Source: three-view drawing plus pictorial views. Frame: mm from the lowest corner of the part. Coordinates: 2 decimals unless noted, no trailing zeros. Write each loop counter-clockwise with the first axis right and the second up, starting at its lowest first coordinate (ties: lowest second). Pieces come first, ordered by that corner, then holes. Notation, with made-up numbers: (-25.5, 51.5) -> (23.5, 51.5) arc R19 ccw to (23.5, 69.5) -> close; hole circle Ø8 at (-27, 85.5). An arc over 180 degrees is marked (long way). One line per item, written item: value. Start each with the question number.
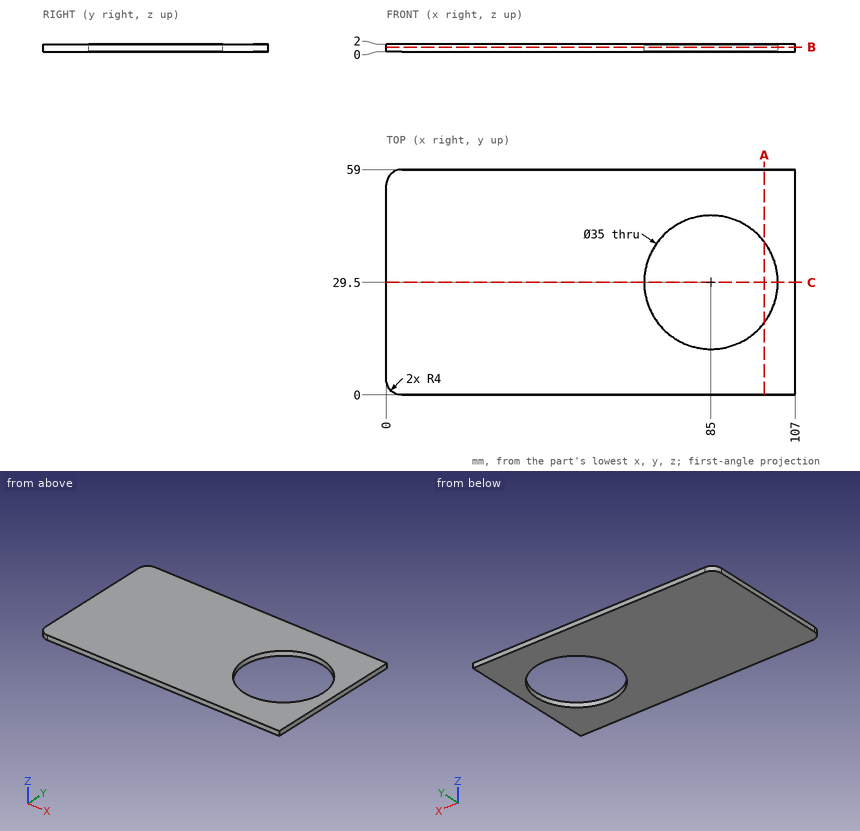
Q1. Cut plane A-A on x = 99. Output: boundary loops of the cut face in (y, z).
Q2. Cut plane C-C on y = 29.5. Output: boundary loops of the cut face in (x, z).
Q3. Line query: L1, parallel to Y at x = 85, z = 1.2; L2, parallel to X at y = 18, z = 1.45; L3, parallel to X at y = 20, z = 1.8. Output: solid intervals per line, ascending. Write a range as from..to.
Q4. First-contact query: P1, Ø3, axis at x = 56, y = 21, coming from the -Z side. Flat tip, straight axial feed; report the tip coordinate or a pass-through.
Q5. Cut plane B-B on z = 1.2. Output: boundary loops of the cut face in (x, y).
Solution:
1. outline: (0, 0) -> (19, 0) -> (19, 2) -> (0, 2) -> close; (40, 0) -> (59, 0) -> (59, 2) -> (40, 2) -> close
2. outline: (0, 0) -> (67.5, 0) -> (67.5, 2) -> (0, 2) -> close; (102.5, 0) -> (107, 0) -> (107, 2) -> (102.5, 2) -> close
3. L1: 0..12, 47..59
3. L2: 0..71.81, 98.19..107
3. L3: 0..70.3, 99.7..107
4. P1: z = 0
5. outline: (0, 4) arc R4 ccw to (4, 0) -> (107, 0) -> (107, 59) -> (4, 59) arc R4 ccw to (0, 55) -> close; hole circle Ø35 at (85, 29.5)
